from build123d import *

# Parameters (mm, degrees)
F0_R      = 15
F1_DEPTH  = 2
F2_R      = 17
F2_R_2    = 15
F3_DEPTH  = 1.5
F4_R      = 17
F4_R_2    = 15
F5_DEPTH  = 1.5
F6_R      = 1.27
F7_R      = 9.5
F8_DEPTH  = 9
F9_R      = 9.5
F10_DEPTH = 9
F11_R     = 7.5
F12_DEPTH = 22
F13_R     = 0.762


# Not quite as in the source:
# - a fillet or chamfer that OpenCascade refuses, or shapes differently, is made with other operations: its cross-section is extruded or revolved along the edge and cut away or added
# - a pattern or mirror of a feature is missing from the dataset's text; its kind, count and spacing are read off the source's solid


with BuildPart() as f1:
    # F0 (on Front) → F1 (new body)
    with BuildSketch(Plane.XZ):
        Circle(F0_R)
    extrude(amount=F1_DEPTH)

    # F2 (on face) → F3 (join)
    with BuildSketch(Plane.XZ.offset(2)):
        Circle(F2_R)
        Circle(F2_R_2, mode=Mode.SUBTRACT)
        Circle(F2_R_2)
    f3 = extrude(amount=F3_DEPTH)

    # F3_copies: F3 across plane
    add(f3.mirror(Plane.ZX.offset(-1)))

    # F4 (on face) → F5 (join)
    with BuildSketch(Plane(origin=(0, 0, 0), x_dir=(-1, 0, 0), z_dir=(0, 1, 0))):
        Circle(F4_R)
        Circle(F4_R_2, mode=Mode.SUBTRACT)
    extrude(amount=F5_DEPTH)

    # F6
    f6_edges = [f1.edges().sort_by_distance(p)[0] for p in [
        (-17, -3.5, 0),
        (-17, 1.5, 0),
    ]]
    fillet(f6_edges, radius=F6_R)

    # F7 (on face) → F8 (join)
    with BuildSketch(Plane.XZ.offset(3.5)):
        Circle(F7_R)
    extrude(amount=F8_DEPTH)

    # F9 (on face) → F10 (join)
    with BuildSketch(Plane(origin=(0, 1.5, 0), x_dir=(-1, 0, 0), z_dir=(0, 1, 0))):
        Circle(F9_R)
    extrude(amount=F10_DEPTH)

    # F11 (on face) → F12 (cut)
    with BuildSketch(Plane.XZ.offset(12.5)):
        Circle(F11_R)
    extrude(amount=-F12_DEPTH, mode=Mode.SUBTRACT)

    # F13
    f13_edges = [f1.edges().sort_by_distance(p)[0] for p in [
        (-7.5, 9.5, 0),
    ]]
    fillet(f13_edges, radius=F13_R)

    # F14: fillet of radius 5.08 on 1 edges, made by hand

    # F14_s1 → F14_t2 (revolve, cut)
    with BuildSketch(Plane.XY):
        with BuildLine():
            ThreePointArc((7.5, -12.5), (8.9726256161, -10.7140835586), (9.5, -8.4601980247))
            Line((9.5, -8.4601980247), (9.5, -12.5))
            Line((9.5, -12.5), (7.5, -12.5))
        make_face()
    revolve(axis=Axis((0, -12.5, 0), (0, -1, 0)), mode=Mode.SUBTRACT)


solid = f1.part
For this review, take the finished solid that the model builds, in its own axes (mm). A direction names the side the tool comes from. Round coordinates to 2 decimals unless told otherwise and drop trailing zeros. Loops run counter-clockwise (first coordinate to the right, second up) from the corner with the lowest first, then second, coordinate; pieces in that order, holes last. Notation, with made-up numbers: (8, 13.5) - (44, 13.5) arc R23 ccw to (44, 50.5) - close; hole circle Ø4 at (35, -28). An arc over 180 degrees is marked (long way). Use one line per item in the form item = value.
1) Mouldability with a two-part tool opening along Z and no side actions: class faces 1 (the face through (6, -2, -14)), 2 (the face through (-14.985, -0.986, 0.66)), 3 (the face through (0, 9.5, 0)) as pulls with the +Z half, pulls with the -Z half, needs draft (parallel to the pull), parting line crosses it, or undercut.
Solutions:
face_1 = needs draft
face_2 = parting line crosses it
face_3 = undercut
2) Wall thickness on probe 1 along Z at (x, y) = (0, 3.5); probe 2 along Y at (x, z) = (-4, -11.5); probe 3 along Z at (x, y) = (0, -0.25): over which ranges is each line inside the solid? List them lowest first.
Solutions:
probe_1 = -9.5 to -7.5, 7.5 to 9.5
probe_2 = -3.5 to 1.5
probe_3 = -15 to -7.5, 7.5 to 15
3) We need section B-B on y = -0.5. Write out the cut boundary in (x, z), then the cut area to 3 significant figures.
Solutions:
outline = circle Ø30 at (0, 0); hole circle Ø15 at (0, 0)
area = 530 mm2
4) Tool access review of faces 4 (the face through (6, 0, -14)), 5 (the face through (7, 1.5, -7)), 6 (the face through (0, 10.5, 0)), 7 (the face through (7, -3.5, -7)): name each direction out of +Z, -Z, +X, -X, +Y, -Y from which nothing blocks a thin tool from reaching the whole face with its end or side.
Solutions:
face_4 = none
face_5 = +Y
face_6 = +Z, -Z, +X, -X, +Y
face_7 = -Y
5) Clearance check with flat-ended pins moving along their axes: P1, Ø12, axis at y = -1.5, z = 10, coming from the -X side; P2, Ø12, axis at x = 0, z = 0, coming from the -Y side; P3, Ø2, axis at y = -3.5, z = -2, coming from the -X side; P4, Ø5, axis at x = -13, y = 7, coming from the +Z side. State where each tip first meets the part, or that it passes through.
Solutions:
P1 = -16.52
P2 = 9.5
P3 = -16.88
P4 = through
6) We need section A-A on y = 5.25. Write out the cut boundary in (x, z).
Solutions:
outline = circle Ø19 at (0, 0); hole circle Ø15 at (0, 0)
